Geometry: see drawing. Coordinates: mm, zero at the bounding-box minimum. A direction names the side the tool comes from. Round coordinates to 2 decimals unless told otherwise and drop trailing zeros. Loops run counter-clockwise (first coordinate to the right, second up) from the corner with the lowest first, then second, coordinate; pieces in that order, holes last. Notation, with made-up numbers: M 24.25,72.5 L 41.25,72.5 A5 ccw 41.25,78.5 Z; hole C 2.25,-5 d7. An arc over 180 degrees is marked long. Answer as a JSON object with one key per item and string values.
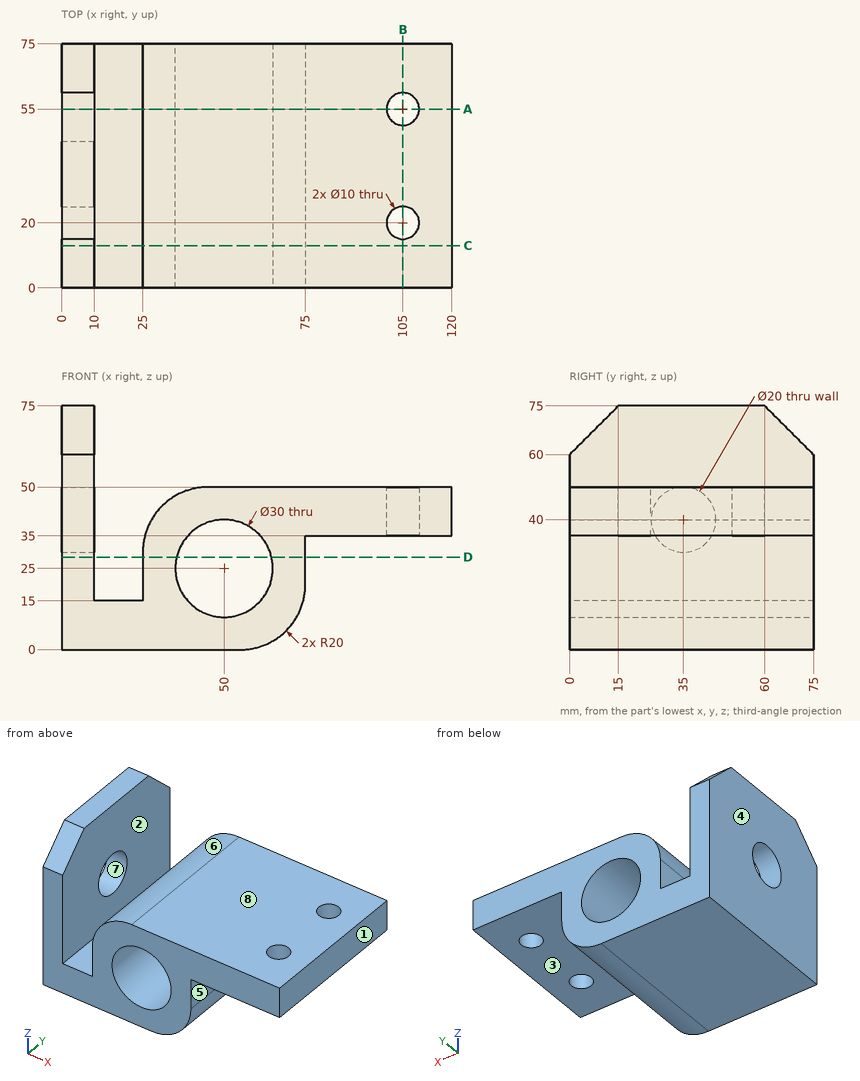
1) Section query A-A (y = 55). Return the cut outline in (x, z), and give its area (3 significant figures).
Results:
{"outline": "M 0,0 L 55,0 A20 ccw 75,20 L 75,35 L 100,35 L 100,50 L 45,50 A20 ccw 25,30 L 25,15 L 10,15 L 10,75 L 0,75 Z; M 110,35 L 120,35 L 120,50 L 110,50 Z; hole C 50,25 d30", "area": "3,120 mm2"}
2) Section query C-C (y = 13). Return the cut outline in (x, z).
Results:
{"outline": "M 0,0 L 55,0 A20 ccw 75,20 L 75,35 L 120,35 L 120,50 L 45,50 A20 ccw 25,30 L 25,15 L 10,15 L 10,73 L 0,73 Z; hole C 50,25 d30"}
3) Section query D-D (z = 28.5). Return the cut outline in (x, y).
Results:
{"outline": "M 0,0 L 10,0 L 10,75 L 0,75 Z; M 25,0 L 35.41,0 L 35.41,75 L 25,75 Z; M 64.59,0 L 75,0 L 75,75 L 64.59,75 Z"}
4) Reachability of the marked faces 5, 6, 7 and 8 from +Z, -Z, +X, -X, +Y, -Y: full face, straight path, thin tool, end or side. Return the list, or none.
Results:
{"face 5": "-Z, +X, +Y, -Y", "face 6": "+Z, +Y, -Y", "face 7": "-X", "face 8": "+Z, +X, +Y, -Y"}
5) Pin query (flat end, axial travel): P1, Ø7.5, axis at y = 40, z = 28.5, coming from the +X side; P2, Ø10, axis at x = 65, y = 60.5, coming from the +Z side; P3, Ø6, axis at x = 105, y = 20, coming from the -Z side. Return the tip coordinate at first contact, or that it passes through.
Results:
{"P1": "x = 75", "P2": "z = 50", "P3": "through"}
6) Pull-direction query (X, two-part tool) for the marked faces 1, 2, 3 and 4; classes: +X half, -X half, draft (parallel to the pull), parting line (faces both ways), or undercut.
Results:
{"face 1": "+X half", "face 2": "undercut", "face 3": "draft", "face 4": "-X half"}
7) Section query B-B (x = 105). Return the cut outline in (y, z), and give its area (3 significant figures).
Results:
{"outline": "M 0,35 L 15,35 L 15,50 L 0,50 Z; M 25,35 L 50,35 L 50,50 L 25,50 Z; M 60,35 L 75,35 L 75,50 L 60,50 Z", "area": "825 mm2"}
8) Ray query, line 1 (Y direction, x = 105, z = 39.5); line 2 (X direction, y = 68, z = 28); line 3 (Z direction, x = 4, y = 35). Return the intervals inside material, ascending.
Results:
{"line 1": "0 to 15, 25 to 50, 60 to 75", "line 2": "0 to 10, 25 to 35.3, 64.7 to 75", "line 3": "0 to 30, 50 to 75"}
